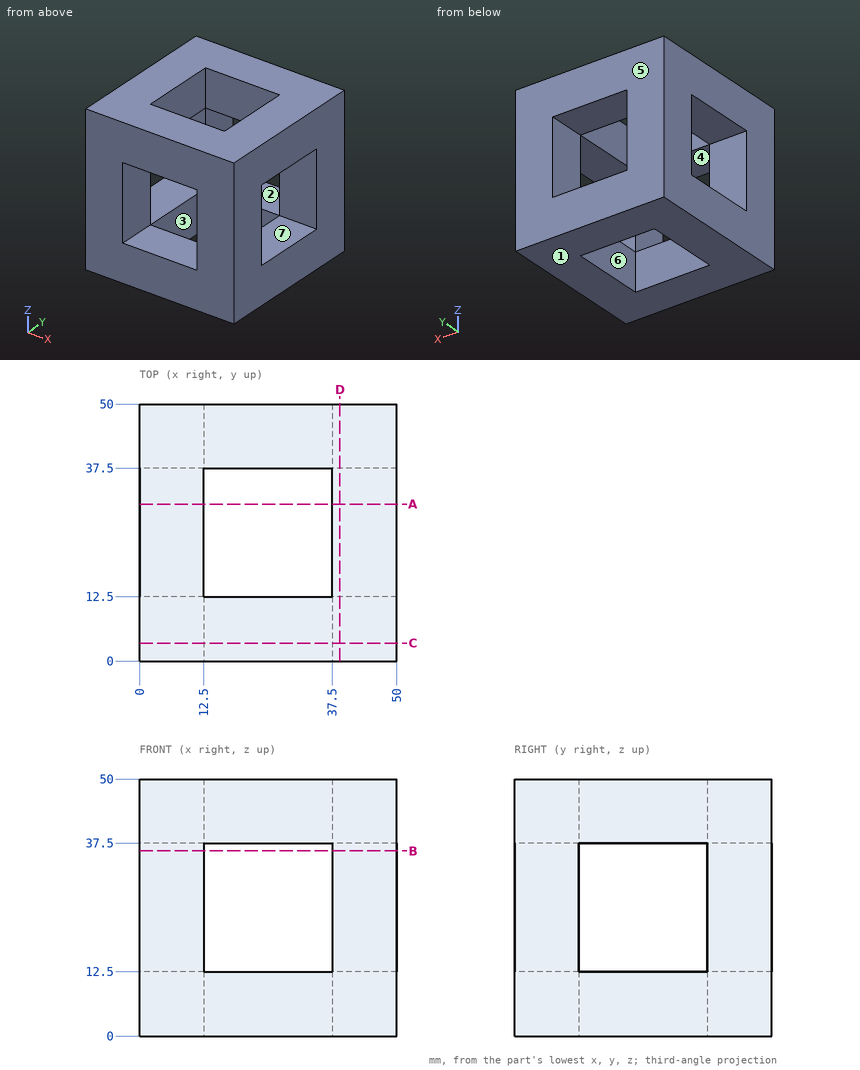
Print and shaded views of the part. All mm, measured from the part's lowest x, y and z. A direction names the side the tool comes from. Round coordinates to 2 decimals unless told otherwise and drop trailing zeros. Order: outer loops, then holes, each group sorted by start corner. A loop starts at its lowest first (then second) coordinate and runs counter-clockwise, first axis right, second up.
Q1. Two-plate mould, pull along Z, no slides. Class the marked faces 1, 2 and 3: pulls with the +Z half, pulls with the -Z half, needs draft (parallel to the pull), parting line crosses it, or undercut.
Q2. Which spindle directions (+Z, -Z, +X, -X, +Y, -Y) get a long thin tool onto all of the face, cutting with end or side? Do the marked faces 4, 5, 6 and 7. Say none if no direction does.
Q3. Wall check: L1, parallel to X at y = 42.5, z = 32.5. Give the ranges that are in metal, low to high.
Q4. Slice it at A-A (y = 30.5). Write the cut outline in (x, z).
Q5. Slice it at C-C (y = 3.5). Write the cut outline in (x, z).
Results below:
1. face 1: pulls with the -Z half
1. face 2: undercut
1. face 3: needs draft
2. face 4: +Y, -Y
2. face 5: +Z, -Z, +X, -X, +Y
2. face 6: +Z, -Z
2. face 7: +X, -X
3. L1: x = 0 to 12.5, 37.5 to 50
4. outline: (0, 0) - (12.5, 0) - (12.5, 12.5) - (0, 12.5) - close; (0, 37.5) - (12.5, 37.5) - (12.5, 50) - (0, 50) - close; (37.5, 0) - (50, 0) - (50, 12.5) - (37.5, 12.5) - close; (37.5, 37.5) - (50, 37.5) - (50, 50) - (37.5, 50) - close
5. outline: (0, 0) - (50, 0) - (50, 50) - (0, 50) - close; hole (12.5, 12.5) - (37.5, 12.5) - (37.5, 37.5) - (12.5, 37.5) - close
